from build123d import *

# Parameters (mm, degrees)
ESQUISSE1_W      = 70
ESQUISSE1_H      = 40
EXTRUSION1_DEPTH = 15
CONG_1_R         = 2
ESQUISSE2_R      = 1.5
ESQUISSE2_R_2    = 0.75
EXTRUSION2_DEPTH = 5


with BuildPart() as part:
    # Esquisse1 → Extrusion1 (new body)
    with BuildSketch(Plane(origin=(0, 0, 0), x_dir=(1, 0, 0), z_dir=(0, 1, 0))):
        with Locations((35, 20)):
            Rectangle(ESQUISSE1_W, ESQUISSE1_H)
    extrude(amount=EXTRUSION1_DEPTH)

    # Congé1
    cong_1_edges = [part.edges().sort_by_distance(p)[0] for p in [
        (70, 15, -20),
        (35, 15, -40),
        (0, 15, -20),
        (35, 0, -40),
        (70, 0, -20),
        (35, 0, 0),
        (0, 0, -20),
        (35, 15, 0),
        (0, 7.5, -40),
        (70, 7.5, -40),
        (70, 7.5, 0),
        (0, 7.5, 0),
    ]]
    fillet(cong_1_edges, radius=CONG_1_R)

    # Esquisse2 → Extrusion2 (add)
    with BuildSketch(Plane(origin=(70, 0, 0), x_dir=(0, 0, -1), z_dir=(1, 0, 0))):
        with Locations(Location((6, 7.5, 0), (0, 0, 180))):
            Circle(ESQUISSE2_R)
        with Locations(Location((10, 7.5, 0), (0, 0, 180))):
            Circle(ESQUISSE2_R)
        with Locations(Location((30, 7.5, 0), (0, 0, 180))):
            Circle(ESQUISSE2_R_2)
        with Locations(Location((32, 7.5, 0), (0, 0, 180))):
            Circle(ESQUISSE2_R_2)
        with Locations(Location((34, 7.5, 0), (0, 0, 180))):
            Circle(ESQUISSE2_R_2)
    extrude(amount=EXTRUSION2_DEPTH)


solid = part.part
The model under review builds one solid part; all positions refer to its coordinate system, in mm. A direction names the side the tool comes from. Round coordinates to 2 decimals unless told otherwise and drop trailing zeros. Loops run counter-clockwise (first coordinate to the right, second up) from the corner with the lowest first, then second, coordinate; pieces in that order, holes last. Notation, with made-up numbers: (-39, 83) -> (-33, 83) arc R15 ccw to (-33, 109) -> close; hole circle Ø6 at (64, -39). An arc over 180 degrees is marked (long way). Answer as CSV lines item,"result".
1) Add section B-B on z = -30. Write out the cut boundary in (x, y).
Geometry results:
outline,"(0, 2) arc R2 ccw to (2, 0) -> (68, 0) arc R2 ccw to (70, 2) -> (70, 6.75) -> (75, 6.75) -> (75, 8.25) -> (70, 8.25) -> (70, 13) arc R2 ccw to (68, 15) -> (2, 15) arc R2 ccw to (0, 13) -> close"
2) Add section C-C on x = 69. Write out the cut boundary in (y, z).
Geometry results:
outline,"(0.27, -38) arc R1.73 ccw to (2, -39.73) -> (13, -39.73) arc R1.73 ccw to (14.73, -38) -> (14.73, -2) arc R1.73 ccw to (13, -0.27) -> (2, -0.27) arc R1.73 ccw to (0.27, -2) -> close"
3) Add section D-D on z = -10. Write out the cut boundary in (x, y), plus the area to 3 significant figures.
Geometry results:
outline,"(0, 2) arc R2 ccw to (2, 0) -> (68, 0) arc R2 ccw to (70, 2) -> (70, 6) -> (75, 6) -> (75, 9) -> (70, 9) -> (70, 13) arc R2 ccw to (68, 15) -> (2, 15) arc R2 ccw to (0, 13) -> close"
area,"1,060 mm²"
4) For P1, Ø1.5, axis at y = 7, z = -18.5, coming from the +X side, flat-tipped, find the tip position at first contact; note if it passes through.
Geometry results:
P1,"stops at x = 70"
5) To check wall thickness, follow line 1 along X through (y, z) = (5.75, -7); line 2 along Z through (x, y) = (57, 13.5); line 3 along Z through (x, y) = (28.5, 14). State the ranges of each line that lie inside material, in increasing order. Write a range as from..to.
Geometry results:
line 1,"x = 0..70"
line 2,"z = -39.94..-0.06"
line 3,"z = -39.73..-0.27"
6) Draft analysis for pull direction Z (two halves, no side actions). For faces 3 (the face through (35.46, 14.4, -0.57)), 4 (the face through (75, 7, -30)), 5 (the face through (72.465, 7.275, -31.285)), state which applies: pulls with the +Z half, pulls with the -Z half, needs draft (parallel to the pull), parting line crosses it, or undercut.
Geometry results:
face 3,"pulls with the +Z half"
face 4,"needs draft"
face 5,"undercut"
7) Add section A-A on y = 7.5. Write out the cut boundary in (x, z).
Geometry results:
outline,"(0, -38) arc R2 ccw to (2, -40) -> (68, -40) arc R2 ccw to (70, -38) -> (70, -34.75) -> (75, -34.75) -> (75, -33.25) -> (70, -33.25) -> (70, -32.75) -> (75, -32.75) -> (75, -31.25) -> (70, -31.25) -> (70, -30.75) -> (75, -30.75) -> (75, -29.25) -> (70, -29.25) -> (70, -11.5) -> (75, -11.5) -> (75, -8.5) -> (70, -8.5) -> (70, -7.5) -> (75, -7.5) -> (75, -4.5) -> (70, -4.5) -> (70, -2) arc R2 ccw to (68, 0) -> (2, 0) arc R2 ccw to (0, -2) -> close"
8) Tool access review of faces 1 (the face through (35, 15, -20)), 2 (the face through (72.465, 7.275, -29.285)): name each direction out of +Z, -Z, +X, -X, +Y, -Y from which nothing blocks a thin tool from reaching the whole face with its end or side.
Geometry results:
face 1,"+Z, -Z, +X, -X, +Y"
face 2,"+X"
